```python
from build123d import *

# Parameters (mm, degrees)
F1_DEPTH = 10
F2_R     = 2.5
F3_DEPTH = 5
F4_R     = 2.5
F5_DEPTH = 5
F6_R     = 2


with BuildPart() as f1:
    # F0 (on Right) → F1 (new body)
    with BuildSketch(Plane.YZ):
        Polygon((-30, 0), (20, 0), (20, 5), (-25, 5), (-25, 46), (5, 46), (5, 200), (0, 200), (0, 50), (-30, 50), align=None)
    extrude(amount=F1_DEPTH)

    # F2 (on face) → F3 (cut, through all)
    with BuildSketch(Plane.XZ):
        with BuildLine():
            ThreePointArc((2.5, 200), (5, 197.5), (7.5, 200))
            Line((7.5, 200), (2.5, 200))
        make_face()
        with Locations((5, 60)):
            Circle(F2_R)
    extrude(amount=-F3_DEPTH, mode=Mode.SUBTRACT)

    # F4 (on face) → F5 (cut, through all)
    with BuildSketch(Plane(origin=(0, 0, 0), x_dir=(1, 0, 0), z_dir=(0, 0, -1))):
        with Locations((5, 20)):
            Circle(F4_R)
        with Locations((5, 5)):
            Circle(F4_R)
        with Locations((5, -10)):
            Circle(F4_R)
    extrude(amount=-F5_DEPTH, mode=Mode.SUBTRACT)

    # F6
    f6_edges = [f1.edges().sort_by_distance(p)[0] for p in [
        (5, -30, 50),
        (5, -25, 46),
        (5, -30, 0),
        (5, -25, 5),
        (5, 5, 46),
        (5, 0, 50),
        (1.25, 5, 200),
        (8.75, 5, 200),
        (1.25, 0, 200),
        (8.75, 0, 200),
    ]]
    fillet(f6_edges, radius=F6_R)


solid = f1.part
```
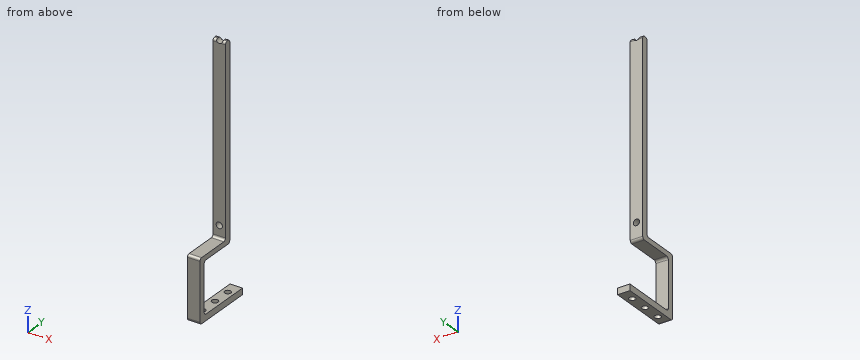
The model under review builds one solid part; all positions refer to its coordinate system, in mm. Coordinates: 2 decimals unless noted, no trailing zeros. Order: outer loops, then holes, each group sorted by start corner. A loop starts at its lowest first (then second) coordinate and runs counter-clockwise, first axis right, second up. Notation, with made-up numbers: (44, 21) -> (57, 21) arc R16 cw to (57, 33) -> close; hole circle Ø2 at (77, 30). An arc over 180 degrees is marked (long way). Answer in a Markdown table with one row per item. Add a question column.
Item 1: We need section D-D on z = 80.5. Write out the cut boundary in (x, y).
Item 2: Clearance check with flat-ended pins moving along their axes: pin 1 (4 mm diameter, centred on x = 5, y = -5, fed in from +Z); pin 2 (3 mm diameter, centred on x = 6, z = 132.5, fed in from +Y); pin 3 (3 mm diameter, centred on x = 2.5, z = 20.5, fed in from +Y). State where each tip first meets the part, or that it passes through.
Item 3: We need section A-A on y = 10. Write out the cut boundary in (x, z).
Item 4: We need section B-B on y = -20. Write out the cut boundary in (x, z), plus the area to 3 significant figures.
Item 5: To check wall thickness, follow probe 1 along Z at (x, y) = (5, -17); probe 2 along X at (y, z) = (-20, 2.65); probe 3 along Z at (x, y) = (3.5, 7). State the ranges of each line that lie inside material, in increasing order.
Final values:
| question | item | result |
|---|---|---|
| 1 | outline | (0, 0) -> (10, 0) -> (10, 5) -> (0, 5) -> close |
| 2 | pin 1 | stops at z = 50 |
| 2 | pin 2 | stops at y = 5 |
| 2 | pin 3 | stops at y = -25 |
| 3 | outline | (0, 0) -> (2.5, 0) -> (2.5, 5) -> (0, 5) -> close; (7.5, 0) -> (10, 0) -> (10, 5) -> (7.5, 5) -> close |
| 4 | outline | (0, 0) -> (2.5, 0) -> (2.5, 5) -> (0, 5) -> close; (0, 46) -> (10, 46) -> (10, 50) -> (0, 50) -> close; (7.5, 0) -> (10, 0) -> (10, 5) -> (7.5, 5) -> close |
| 4 | area | 65.0 mm2 |
| 5 | probe 1 | z = 0 to 5, 46 to 50 |
| 5 | probe 2 | x = 0 to 2.5, 7.5 to 10 |
| 5 | probe 3 | z = 0 to 5 |
